```python
from build123d import *

# Parameters (mm, degrees)
F0_W      = 370
F0_H      = 400
F1_DEPTH  = 12
F2_W      = 10
F2_H      = 75
F3_DEPTH  = 25
F4_R      = 1
F5_DEPTH  = 5
F6_R      = 1
F7_DEPTH  = 25
F8_R      = 1
F9_DEPTH  = 25
F10_R     = 1
F11_DEPTH = 5
F12_R     = 1
F13_DEPTH = 5
F14_R     = 1
F15_DEPTH = 5


with BuildPart() as f1:
    # F0 (on Top) → F1 (new body)
    with BuildSketch(Plane.XY):
        Rectangle(F0_W, F0_H)
    extrude(amount=F1_DEPTH)

    # F2 (on face) → F3 (cut)
    with BuildSketch(Plane.XY.offset(12)):
        with Locations((-5, -117.5)):
            Rectangle(F2_W, F2_H)
    extrude(amount=-F3_DEPTH, mode=Mode.SUBTRACT)

    # F4 (on face) → F5 (cut)
    with BuildSketch(Plane.XY.offset(12)):
        with Locations((-50, -80)):
            Circle(F4_R)
        with Locations((-15, -80)):
            Circle(F4_R)
        with Locations((-50, -140)):
            Circle(F4_R)
        with Locations((-30, -50)):
            Circle(F4_R)
        with Locations((-50, -50)):
            Circle(F4_R)
    extrude(amount=-F5_DEPTH, mode=Mode.SUBTRACT)

    # F6 (on face) → F7 (cut)
    with BuildSketch(Plane.XY.offset(12)):
        with Locations((-175, -10)):
            Circle(F6_R)
        with Locations((-175, 10)):
            Circle(F6_R)
    extrude(amount=-F7_DEPTH, mode=Mode.SUBTRACT)

    # F8 (on face) → F9 (cut)
    with BuildSketch(Plane.XY.offset(12)):
        with Locations((175, 10)):
            Circle(F8_R)
        with Locations((175, -10)):
            Circle(F8_R)
    extrude(amount=-F9_DEPTH, mode=Mode.SUBTRACT)

    # F10 (on face) → F11 (cut)
    with BuildSketch(Plane.XY.offset(12)):
        with Locations((60, 20)):
            Circle(F10_R)
        with Locations((-10, -20)):
            Circle(F10_R)
    extrude(amount=-F11_DEPTH, mode=Mode.SUBTRACT)

    # F12 (on face) → F13 (cut)
    with BuildSketch(Plane.XY.offset(12)):
        with Locations((115, -15)):
            Circle(F12_R)
        with Locations((115, -30)):
            Circle(F12_R)
    extrude(amount=-F13_DEPTH, mode=Mode.SUBTRACT)

    # F14 (on face) → F15 (cut)
    with BuildSketch(Plane.XY.offset(12)):
        with Locations((115, 30)):
            Circle(F14_R)
        with Locations((115, 15)):
            Circle(F14_R)
    extrude(amount=-F15_DEPTH, mode=Mode.SUBTRACT)


solid = f1.part
```
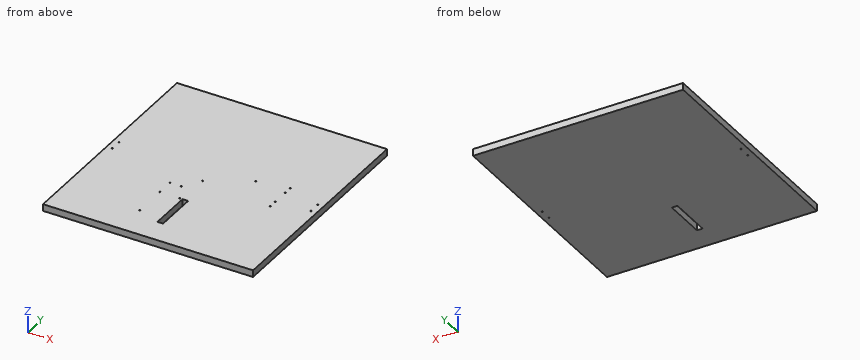
Source: CAD feature listing. Evaluate the final solid. Frame: model axes, mm. Round coordinates to 2 decimals unless told otherwise and drop trailing zeros. Loops run counter-clockwise (first coordinate to the right, second up) from the corner with the lowest first, then second, coordinate; pieces in that order, holes last. Notation, with made-up numbers: M 25.5,-0.5 L 82.5,-0.5 A19 cw 82.5,4.5 Z; hole C 72,-21.75 d6. An arc over 180 degrees is marked long. Use a Markdown table: item, result. Add a question column.
1. Ray query, line 1 along Y through (x, z) = (175, 7.5); line 2 along Y through (x, z) = (115, 9.55); line 3 along Y through (x, z) = (-50, 10.3). Return the intervals inside material, ascending. Write a range as [from, to].
2. Cut plane A-A, the plane y = -93. Output: boundary loops of the cut face in (x, z), and give its area (3 significant figures).
3. Contact query for a flat-ended pin moving along its axis: pin 1 (2.5 mm diameter, centred on x = 115, y = -15, fed in from -Z). Output: stop coordinate, or through.
Solution:
| question | item | result |
|---|---|---|
| 1 | line 1 | y = [-200, -11], [-9, 9], [11, 200] |
| 1 | line 2 | y = [-200, -31], [-29, -16], [-14, 14], [16, 29], [31, 200] |
| 1 | line 3 | y = [-200, -141], [-139, -81], [-79, -51], [-49, 200] |
| 2 | outline | M -185,0 L -10,0 L -10,12 L -185,12 Z; M 0,0 L 185,0 L 185,12 L 0,12 Z |
| 2 | area | 4,320 mm2 |
| 3 | pin 1 | stops at z = 0 |
